Here's how the part is built. I have some questions about the finished solid (model axes, mm). A direction names the side the tool comes from. Round coordinates to 2 decimals unless told otherwise and drop trailing zeros. Write each loop counter-clockwise with the first axis right and the second up, starting at its lowest first coordinate (ties: lowest second). Pieces come first, ordered by that corner, then holes. Notation, with made-up numbers: (51.5, 60) -> (69.5, 60) arc R4 ccw to (69.5, 67) -> close; hole circle Ø5 at (4, 81.5). An arc over 180 degrees is marked (long way). Put each result on its own line as item: value. Start each with the question number.
1. I need wall thicknesses on probe 1 along X at (y, z) = (2.35, 1); probe 2 along Z at (x, y) = (6.5, 3.2); probe 3 along Z at (x, y) = (6.75, 3.8). Which ranges of each line are inside material? Lowest first, please. Write a range as from..to.
2. We'd pull the mould along Z, two halves only. Please class faces 1 (the face through (7.2, 2.46, -17.73)), 2 (the face through (6.873, 2.465, 15.266)), 3 (the face through (7.17, 1.48, -16.23)): +Z half, -Z half, draft (parallel to the pull), parting line (faces both ways), or undercut.
3. For pin 1 (4 mm diameter, centred on x = 7.04, z = 5.77, fed in from +Y); pin 2 (5 mm diameter, centred on x = 4, z = 7, fed in from -Y), each with a flat end and sliding along its axis, tell me the tip position at first contact or that it passes through.
4. Which directions (+Z, -Z, +X, -X, +Y, -Y) give clear straight access to the entire face, cutting with the end or side of a thin tool? Please do faces 4 (the face through (7.52, 4.01, 11.92)), 5 (the face through (6.905, 1.479, 13.767)).
5. Suppose I cut it at C-C (x = 6.25). Please give me the cut outline in (y, z).
6. Suppose I cut it at A-A (z = 6.5). Please give me the cut outline in (x, y).
7. Suppose I cut it at D-D (z = -3). Please give me the cut outline in (x, y), then the cut area to 3 significant figures.
8. Suppose I cut it at B-B (y = 2.25). Please give me the cut outline in (x, z), then the cut area to 3 significant figures.
```python
from build123d import *

# Parameters (mm, degrees)
BOSS_EXTRUDE2_DEPTH     = 5
CUT_EXTRUDE2_DEPTH      = 3
CUT_EXTRUDE3_DEPTH      = 24.124843106
CUT_EXTRUDE3_DEPTH_BACK = 3
SKETCH4_R               = 1.25


with BuildPart() as part:
    # Sketch3 → Boss-Extrude2 (new body)
    with BuildSketch(Plane(origin=(0, 0, 0), x_dir=(1, 0, 0), z_dir=(0, 1, 0))):
        with BuildLine():
            Line((-0.462577175, 10.231940285), (-0.462577175, -7.768059715))
            ThreePointArc((-0.462577175, -7.768059715), (7.037422825, -15.268059715), (14.537422825, -7.768059715))
            Line((14.537422825, -7.768059715), (14.537422825, 10.231940285))
            ThreePointArc((14.537422825, 10.231940285), (7.037422825, 17.731940285), (-0.462577175, 10.231940285))
        make_face()
    extrude(amount=BOSS_EXTRUDE2_DEPTH)

    # Sketch2 → Cut-Extrude2 (cut)
    with BuildSketch(Plane(origin=(0, 0, 0), x_dir=(1, 0, 0), z_dir=(0, 1, 0))):
        with BuildLine():
            Line((1.037422825, 10.231940285), (1.037422825, -7.768059715))
            ThreePointArc((1.037422825, -7.768059715), (7.037422825, -13.768059715), (13.037422825, -7.768059715))
            Line((13.037422825, -7.768059715), (13.037422825, 10.231940285))
            ThreePointArc((13.037422825, 10.231940285), (7.037422825, 16.231940285), (1.037422825, 10.231940285))
        make_face()
    extrude(amount=CUT_EXTRUDE2_DEPTH, mode=Mode.SUBTRACT)

    # Sketch4 → Cut-Extrude3 (cut, two sides: drawn at the far end of the back side and taken through both)
    with BuildSketch(Plane.XZ.offset(-3).offset(-CUT_EXTRUDE3_DEPTH_BACK)):
        with Locations(Location((7.037422825, 10.768059715, 0), (0, 0, 90))):
            Circle(SKETCH4_R)
        with Locations(Location((7.037422825, 5.768059715, 0), (0, 0, 90))):
            Circle(SKETCH4_R)
    extrude(amount=CUT_EXTRUDE3_DEPTH + CUT_EXTRUDE3_DEPTH_BACK, mode=Mode.SUBTRACT)


solid = part.part
```
Verdict:
1. probe 1: x = -0.46..1.04, 13.04..14.54
1. probe 2: z = -17.71..4.64, 6.9..9.64, 11.9..15.25
1. probe 3: z = -17.73..4.55, 6.98..9.55, 11.98..15.26
2. face 1: -Z half
2. face 2: +Z half
2. face 3: undercut
3. pin 1: stops at y = 5
3. pin 2: stops at y = 3
4. face 4: +Y, -Y
4. face 5: -Y
5. outline: (0, -17.69) -> (5, -17.69) -> (5, 4.8) -> (3, 4.8) -> (3, -16.18) -> (0, -16.18) -> close; (0, 13.72) -> (3, 13.72) -> (3, 11.74) -> (5, 11.74) -> (5, 15.23) -> (0, 15.23) -> close; (3, 6.74) -> (5, 6.74) -> (5, 9.8) -> (3, 9.8) -> close
6. outline: (-0.46, 0) -> (1.04, 0) -> (1.04, 3) -> (6.02, 3) -> (6.02, 5) -> (-0.46, 5) -> close; (8.05, 3) -> (13.04, 3) -> (13.04, 0) -> (14.54, 0) -> (14.54, 5) -> (8.05, 5) -> close
7. outline: (-0.46, 0) -> (1.04, 0) -> (1.04, 3) -> (13.04, 3) -> (13.04, 0) -> (14.54, 0) -> (14.54, 5) -> (-0.46, 5) -> close
7. area: 39.0 mm^2
8. outline: (-0.46, -10.23) arc R7.5 ccw to (14.54, -10.23) -> (14.54, 7.77) arc R7.5 ccw to (-0.46, 7.77) -> close; hole (1.04, -10.23) arc R6 ccw to (13.04, -10.23) -> (13.04, 7.77) arc R6 ccw to (1.04, 7.77) -> close
8. area: 118 mm^2
